Autodesk Fusion 360 part; units mm, degrees
sketch "Right_enclosure_outline" plane through (0, 0, 0) normal (0, 0, 1) x (1, 0, 0)
  line L0 (-73.4538, 34.3576) -> (65.5462, 34.3576)
  arc A0 (-73.5521, 34.3552) -> (-74.4514, 33.4559) centre (-73.4538, 33.3576) ccw
  line L1 (-74.4538, -39.6424) -> (-74.4538, 33.3576)
  line L2 (-58.9585, -65.7908) -> (-74.4538, -39.6424)
  line L3 (-39.4538, -55.6424) -> (-57.5971, -66.1464)
  line L4 (-21.4538, -50.6424) -> (-39.4538, -55.6424)
  arc A1 (-58.9067, -65.8736) -> (-57.6828, -66.1933) centre (-58.0982, -65.2811) ccw
  line L5 (-0.9538, -50.6424) -> (-21.4538, -50.6424)
  arc A2 (-0.8556, -50.64) -> (0.0438, -49.7406) centre (-0.9538, -49.6424) ccw
  line L6 (0.0462, -32.6424) -> (0.0462, -49.6424)
  line L7 (24.5462, -31.6424) -> (1.0462, -31.6424)
  line L8 (25.5462, -34.6424) -> (25.5462, -32.6424)
  line L9 (64.5462, -35.6424) -> (26.5462, -35.6424)
  line L10 (66.5462, 33.3576) -> (66.5462, -33.6424)
  line L11 (2.5, -32.5) -> (22.5, -32.5)
  line L12 (-56.6719, -66.5254) -> (-39.1, -56.2)
  line L13 (-39.1, -56.2) -> (-21.4538, -51.2983)
  line L14 (-21.4538, -51.2983) -> (-1.5, -51.2983)
  arc A3 (22.5, -32.5) -> (24.5, -34.5) centre (22.5, -34.5) cw
  line L15 (24.5, -34.5) -> (24.5, -36.0424)
  line L16 (-74.8538, 31.6376) -> (-74.8538, 0.3904)
  line L17 (-74.8538, 0.3904) -> (-74.8538, -39.752)
  line L18 (-74.8538, 34) -> (-74.8538, 31.6376)
  line L19 (-74.8538, -39.752) -> (-59.4057, -65.8207)
  line L20 (0.5, -49.2983) -> (0.5, -34.5)
  arc A4 (0.5, -34.5) -> (2.5, -32.5) centre (2.5, -34.5) cw
  line L21 (65.0462, 36) -> (-72.8538, 36)
  line L22 (67.0462, -34.0424) -> (67.0462, 34)
  line L23 (44.5449, -36.0424) -> (65.0462, -36.0424)
  line L24 (24.5, -36.0424) -> (44.5449, -36.0424)
  line L25 (-21.4538, -51.2983) -> (-1.5, -51.2983)
  line L26 (2.5, -32.5) -> (22.5, -32.5)
  line L27 (-74.8538, 34) -> (-74.8538, 31.6376)
  arc A5 (67.0462, 34) -> (65.0462, 36) centre (65.0462, 34) ccw
  line L28 (-39.1, -56.2) -> (-21.4538, -51.2983)
  line L29 (0.5, -49.2983) -> (0.5, -34.5)
  line L30 (65.0462, 36) -> (-72.8538, 36)
  line L31 (67.0462, -34.0424) -> (67.0462, 34)
  arc A6 (-72.8538, 36) -> (-74.8538, 34) centre (-72.8538, 34) ccw
  line L32 (-74.8538, 0.3904) -> (-74.8538, -39.752)
  arc A7 (65.0462, -36.0424) -> (67.0462, -34.0424) centre (65.0462, -34.0424) ccw
  line L33 (-56.6719, -66.5254) -> (-39.1, -56.2)
  line L34 (-74.8538, -39.752) -> (-59.4057, -65.8207)
  line L35 (24.5, -34.5) -> (24.5, -36.0424)
  arc A8 (-59.4057, -65.8207) -> (-56.6719, -66.5254) centre (-57.6851, -64.8011) ccw
  arc A9 (-1.5, -51.2983) -> (0.5, -49.2983) centre (-1.5, -49.2983) ccw
  line L36 (44.5449, -36.0424) -> (65.0462, -36.0424)
  line L37 (-74.8538, 31.6376) -> (-74.8538, 0.3904)
  line L38 (24.5, -36.0424) -> (44.5449, -36.0424)
  line L39 (-20.4997, -58.2983) -> (4.5, -58.2983)
  line L40 (-81.8538, -41.6703) -> (-62.3802, -74.532)
  line L41 (7.5, -55.2983) -> (7.5, -39.5)
  arc A10 (-62.3802, -74.532) -> (-58.2795, -75.5891) centre (-59.7994, -73.0026) ccw
  arc A11 (17.5, -40.0424) -> (20.5, -43.0424) centre (20.5, -40.0424) ccw
  line L42 (7.5, -39.5) -> (17.5, -39.5)
  line L43 (-58.2795, -75.5891) -> (-36.3436, -62.6994)
  line L44 (-81.8538, 31.6376) -> (-81.8538, 0.3904)
  line L45 (-81.8538, 0.3904) -> (-81.8538, -41.6703)
  line L46 (74.0462, -40.0424) -> (74.0462, 40)
  arc A12 (74.0462, 40) -> (71.0462, 43) centre (71.0462, 40) ccw
  line L47 (-36.3436, -62.6994) -> (-20.4997, -58.2983)
  line L48 (44.5449, -43.0424) -> (71.0462, -43.0424)
  arc A13 (-78.8538, 43) -> (-81.8538, 40) centre (-78.8538, 40) ccw
  arc A14 (4.5, -58.2983) -> (7.5, -55.2983) centre (4.5, -55.2983) ccw
  arc A15 (71.0462, -43.0424) -> (74.0462, -40.0424) centre (71.0462, -40.0424) ccw
  line L49 (17.5, -39.5) -> (17.5, -40.0424)
  line L50 (-81.8538, 40) -> (-81.8538, 31.6376)
  line L51 (20.5, -43.0424) -> (44.5449, -43.0424)
  line L52 (71.0462, 43) -> (-78.8538, 43)
  circle A16 centre (-78, 39) radius 1.6
  circle A17 centre (-60, -71) radius 1.6
  circle A18 centre (69.7169, -39.1925) radius 1.6
  circle A19 centre (69.6831, 39.8042) radius 1.6
  circle A20 centre (-65.4538, -25.6424) radius 1.5875
  line L53 (-59.5038, -16.8424) -> (-59.5038, -10.8424)
  line L54 (-65.4038, -16.8424) -> (-65.4038, -10.8424)
  circle A21 centre (60.5462, 28.3576) radius 1.5875
  arc A22 (25.5486, -34.7406) -> (26.4479, -35.64) centre (26.5462, -34.6424) ccw
  arc A23 (25.5438, -32.5441) -> (24.6444, -31.6448) centre (24.5462, -32.6424) ccw
  arc A24 (64.6891, -35.6398) -> (66.5436, -33.7853) centre (64.5462, -33.6424) ccw
  arc A25 (66.5438, 33.4559) -> (65.6444, 34.3552) centre (65.5462, 33.3576) ccw
  arc A26 (-72.8538, 36) -> (-74.8538, 34) centre (-72.8538, 34) ccw
  arc A27 (-59.4057, -65.8207) -> (-56.6719, -66.5254) centre (-57.6851, -64.8011) ccw
  arc A28 (-1.5, -51.2983) -> (0.5, -49.2983) centre (-1.5, -49.2983) ccw
  arc A29 (2.5, -32.5) -> (0.5, -34.5) centre (2.5, -34.5) ccw
  arc A30 (24.5, -34.5) -> (22.5, -32.5) centre (22.5, -34.5) ccw
  arc A31 (65.0462, -36.0424) -> (67.0462, -34.0424) centre (65.0462, -34.0424) ccw
  arc A32 (67.0462, 34) -> (65.0462, 36) centre (65.0462, 34) ccw
  dimension "d1" = 2
extrude "Extrude1" add sketch "Right_enclosure_outline" along normal blind 10.5 contours L39 L40 L41 A10 A11 L42 L43 L44 L45 L46 A12 L47 L48 A13 A14 A15 L49 L50 L51 L52
extrude "Extrude2" add sketch "Right_enclosure_outline" along normal blind 2 contours L11 L12 L13 L14 A3 L15 L16 L17 L18 L19 L20 A4 L21 L22 L23 L24 L25 L26 L27 A5 L28 L29 L30 L31 A6 L32 A7 L33 L34 L35 A8 A9 L36 L37 L38 A26 A27 A28 A29 A30 A31 A32 | A20 | A21
sketch "Sketch2" plane through (0, 0, 0) normal (0, 0, 1) x (1, 0, 0)
  circle A0 centre (69.6831, 39.8042) radius 2.75
  circle A1 centre (69.7169, -39.1925) radius 2.75
  circle A2 centre (-60, -71) radius 2.75
  circle A3 centre (-78, 39) radius 2.75
  point P0 (69.6831, 39.8042)
  point P1 (69.7169, -39.1925)
  point P2 (-60, -71)
  point P3 (-78, 39)
  dimension "d6" = 5.5
  dimension "d9" = 5.5
  dimension "d10" = 5.5
  dimension "d11" = 5.5
extrude "Extrude3" cut sketch "Sketch2" along normal blind 3 contours A0
extrude "Extrude4" cut sketch "Sketch2" along normal blind 3 contours A1 | A2 | A3
sketch "Sketch3" plane through (0, 0, 2) normal (0, 0, 1) x (-1, 0, 0)
  line L0 (-24.5, 34.5) -> (-24.5, 36.0424)
  line L1 (-24.5, 36.0424) -> (-65.0462, 36.0424)
  arc A0 (-65.0462, 36.0424) -> (-67.0462, 34.0424) centre (-65.0462, 34.0424) ccw
  line L2 (-67.0462, 34.0424) -> (-67.0462, -34)
  arc A1 (-67.0462, -34) -> (-65.0462, -36) centre (-65.0462, -34) ccw
  line L3 (-65.0462, -36) -> (72.8538, -36)
  arc A2 (72.8538, -36) -> (74.8538, -34) centre (72.8538, -34) ccw
  line L4 (74.8538, -34) -> (74.8538, 39.752)
  line L5 (74.8538, 39.752) -> (59.4057, 65.8207)
  arc A3 (59.4057, 65.8207) -> (56.6719, 66.5254) centre (57.6851, 64.8011) ccw
  line L6 (56.6719, 66.5254) -> (39.1, 56.2)
  line L7 (39.1, 56.2) -> (21.4538, 51.2983)
  line L8 (21.4538, 51.2983) -> (1.5, 51.2983)
  arc A4 (1.5, 51.2983) -> (-0.5, 49.2983) centre (1.5, 49.2983) ccw
  line L9 (-0.5, 49.2983) -> (-0.5, 34.5)
  arc A5 (-2.5, 32.5) -> (-0.5, 34.5) centre (-2.5, 34.5) ccw
  line L10 (-2.5, 32.5) -> (-22.5, 32.5)
  arc A6 (-24.5, 34.5) -> (-22.5, 32.5) centre (-22.5, 34.5) ccw
  circle A7 centre (65.4538, 25.6424) radius 1.5875
  circle A8 centre (-60.5462, -28.3576) radius 1.5875
  circle A9 centre (65.4538, 25.6424) radius 2.45
  circle A10 centre (65.4538, 25.6424) radius 3.45
  circle A11 centre (-60.5462, -28.3576) radius 2.45
  circle A12 centre (-60.5462, -28.3576) radius 3.45
  point P0 (-60.5462, -28.3576)
  dimension "d14" = 4.9
  dimension "d15" = 1
  dimension "d16" = 4.9
  dimension "d17" = 1
extrude "Extrude5" add sketch "Sketch3" along normal blind 4.9 contours A10 | A12
sketch "swopeniing" plane through (-81.8538, 0, 0) normal (-1, 0, 0) x (0, -1, 0)
  line L0 (-40, 0) -> (41.6703, 0)
  line L1 (41.6703, 10.5) -> (-40, 10.5)
  line L2 (-40, 10.5) -> (-40, 0)
  line L3 (41.6703, 0) -> (41.6703, 10.5)
  line L4 (18.0355, 9.995) -> (18.1755, 9.995)
  arc A0 (13.3155, 9.995) -> (13.6755, 10.355) centre (13.3155, 10.355) ccw
  line L5 (11.8255, 9.995) -> (13.1755, 9.995)
  line L6 (17.6755, 12.195) -> (17.6755, 10.355)
  line L7 (18.1755, 9.995) -> (19.5255, 9.995)
  line L8 (13.6755, 10.355) -> (13.6755, 12.195)
  line L9 (19.5255, 12.895) -> (11.8255, 12.895)
  line L10 (13.6755, 12.195) -> (17.6755, 12.195)
  arc A1 (17.6755, 10.355) -> (18.0355, 9.995) centre (18.0355, 10.355) ccw
  line L11 (11.8255, 12.895) -> (11.8255, 9.995)
  line L12 (19.5255, 9.995) -> (19.5255, 12.895)
  line L13 (13.1755, 9.995) -> (13.3155, 9.995)
  line L14 (18.1255, 9.995) -> (13.2255, 9.995)
extrude "Extrude6" cut sketch "swopeniing" against normal blind 20 contours L1 A0 L5 L8 L11 L13 L14 | L1 L4 L6 L7 A1 L12 L14 | L1 A0 L6 L8 A1 L14
sketch "Niceusbopeninig2" plane through (0, 43, 0) normal (0, 1, 0) x (-1, 0, 0)
  line L0 (-71.0462, 0) -> (78.8538, 0)
  line L1 (-71.0462, 10.5) -> (-71.0462, 0)
  line L2 (78.8538, 10.5) -> (-71.0462, 10.5)
  line L3 (78.8538, 0) -> (78.8538, 10.5)
  line L4 (68.0221, 12.5789) -> (68.2393, 12.4584)
  line L5 (68.2393, 12.4584) -> (68.4202, 12.3136)
  line L6 (68.0221, 9.6111) -> (67.7927, 9.5384)
  line L7 (68.7819, 11.4327) -> (68.7819, 10.7693)
  line L8 (68.4202, 12.3136) -> (68.577, 12.1207)
  line L9 (67.7927, 9.5384) -> (67.5393, 9.5145)
  line L10 (68.7579, 11.6741) -> (68.7819, 11.4327)
  line L11 (67.5393, 9.5145) -> (61.085, 9.5145)
  line L12 (59.8424, 11.4327) -> (59.8664, 11.6741)
  line L13 (60.0473, 10.0696) -> (59.9388, 10.2745)
  line L14 (59.9388, 10.2745) -> (59.8664, 10.5159)
  line L15 (60.3853, 9.7316) -> (60.2041, 9.8767)
  line L16 (60.2041, 9.8767) -> (60.0473, 10.0696)
  line L17 (59.8664, 10.5159) -> (59.8424, 10.7693)
  line L18 (59.8424, 10.7693) -> (59.8424, 11.4327)
  line L19 (59.9388, 11.9152) -> (60.0473, 12.1207)
  line L20 (60.2041, 12.3136) -> (60.3853, 12.4584)
  line L21 (67.5393, 12.6755) -> (67.7927, 12.6513)
  line L22 (61.085, 12.6755) -> (67.5393, 12.6755)
  line L23 (60.3853, 12.4584) -> (60.6025, 12.5789)
  line L24 (67.7927, 12.6513) -> (68.0221, 12.5789)
  line L25 (60.6025, 9.6111) -> (60.3853, 9.7316)
  line L26 (68.2393, 9.7316) -> (68.0221, 9.6111)
  line L27 (61.085, 9.5145) -> (60.8316, 9.5384)
  line L28 (60.6025, 12.5789) -> (60.8316, 12.6513)
  line L29 (60.0473, 12.1207) -> (60.2041, 12.3136)
  line L30 (60.8316, 9.5384) -> (60.6025, 9.6111)
  line L31 (68.6853, 10.2745) -> (68.577, 10.0696)
  line L32 (59.8664, 11.6741) -> (59.9388, 11.9152)
  line L33 (68.6853, 11.9152) -> (68.7579, 11.6741)
  line L34 (68.4202, 9.8767) -> (68.2393, 9.7316)
  line L35 (60.8316, 12.6513) -> (61.085, 12.6755)
  line L36 (68.7819, 10.7693) -> (68.7579, 10.5159)
  line L37 (68.577, 10.0696) -> (68.4202, 9.8767)
  line L38 (68.577, 12.1207) -> (68.6853, 11.9152)
  line L39 (68.7579, 10.5159) -> (68.6853, 10.2745)
extrude "Extrude7" cut sketch "Niceusbopeninig2" against normal blind 68 contours L2 L6 L9 L11 L13 L14 L15 L16 L25 L26 L27 L30 L31 L34 L37 L39
The listing builds one solid part. Answer for the finished solid, in the listing's coordinates (mm). A direction names the side the tool comes from. Round coordinates to 2 decimals unless told otherwise and drop trailing zeros. Loops run counter-clockwise (first coordinate to the right, second up) from the corner with the lowest first, then second, coordinate; pieces in that order, holes last.
1) A cutting plane is placed at C-C on y = -71. Determine the outline of the cut face in (x, z), plus the area to 3 significant figures.
Outcome:
outline: (-64.47, 0) - (-62.75, 0) - (-62.75, 3) - (-61.6, 3) - (-61.6, 10.5) - (-64.47, 10.5) - close; (-58.4, 3) - (-57.25, 3) - (-57.25, 0) - (-50.47, 0) - (-50.47, 10.5) - (-58.4, 10.5) - close
area: 107 mm2
2) A cutting plane is placed at B-B on y = -2.5. Determine the outline of the cut face in (x, z).
Outcome:
outline: (-81.85, 0) - (74.05, 0) - (74.05, 10.5) - (67.05, 10.5) - (67.05, 2) - (-74.85, 2) - (-74.85, 10.5) - (-81.85, 10.5) - close
3) For faces 1 (the face through (7.5, -48, 5)), 2 (the face through (74.046, -1, 5)), 3 (the face through (70, 38, 3)), 4 (the face through (-81.854, 0, 5)), 5 (the face through (12, -32.5, 6)), determine the directions among +Z, -Z, +X, -X, +Y, -Y from which every point of the face is accessible in a straight line to the end or side of a thin tool.
Outcome:
face 1: +Z, -Z, -Y
face 2: +Z, -Z, +X, +Y, -Y
face 3: -Z
face 4: +Z, -Z, -X, +Y, -Y
face 5: +Z
4) A cutting plane is placed at A-A on x = 35.5. Determine the outline of the cut face in (y, z), plus the area to 3 significant figures.
Outcome:
outline: (-43.04, 0) - (43, 0) - (43, 10.5) - (36, 10.5) - (36, 2) - (-36.04, 2) - (-36.04, 10.5) - (-43.04, 10.5) - close
area: 291 mm2
5) For a pull along X with two mould halves and no side action, classify faces 6 (the face through (58.21, 29.09, 4.42)), 7 (the face through (61, 28, 2)), 8 (the face through (-3, 43, 5)), 9 (the face through (73.19, -42.14, 5.18)) as released by +X, released by -X, zero draft, split by the parting line, or undercut.
Outcome:
face 6: undercut
face 7: undercut
face 8: zero draft
face 9: released by +X
6) Consider line 1 (X direction, y = -5, z = 8.25); line 2 (Y direction, x = 20.5, z = 4); line 3 (X direction, y = -35, z = 5). Determine where each line is inside the solid, lowest interval first.
Outcome:
line 1: x = -81.85 to -74.85, 67.05 to 74.05
line 2: y = -43.04 to -32.5, 36 to 43
line 3: x = -81.85 to -74.85, 0.5 to 24.5, 66.8 to 74.05
7) A cutting plane is placed at D-D on z = 5. Give the number of separate pieces and of enclosed holes in the cut face, plus the area to 3 significant figures.
Outcome:
separate pieces: 3
enclosed holes: 7
area: 3,510 mm2
8) Given P1, Ø3, axis at x = -19.5, y = -4, coming from the -Z side; P2, Ø4.5, axis at x = 69.68, y = 39.8, coming from the -Z side; P3, Ø3, axis at x = 39, z = 8, coming from the -Y side; P4, Ø7.5, axis at x = 61.5, y = 27, coming from the +Z side, each flat-ended and moving along its own axis, determine where each tip first touches the part or whether it passes through.
Outcome:
P1: stops at z = 0
P2: stops at z = 3
P3: stops at y = -43.04
P4: stops at z = 6.9
